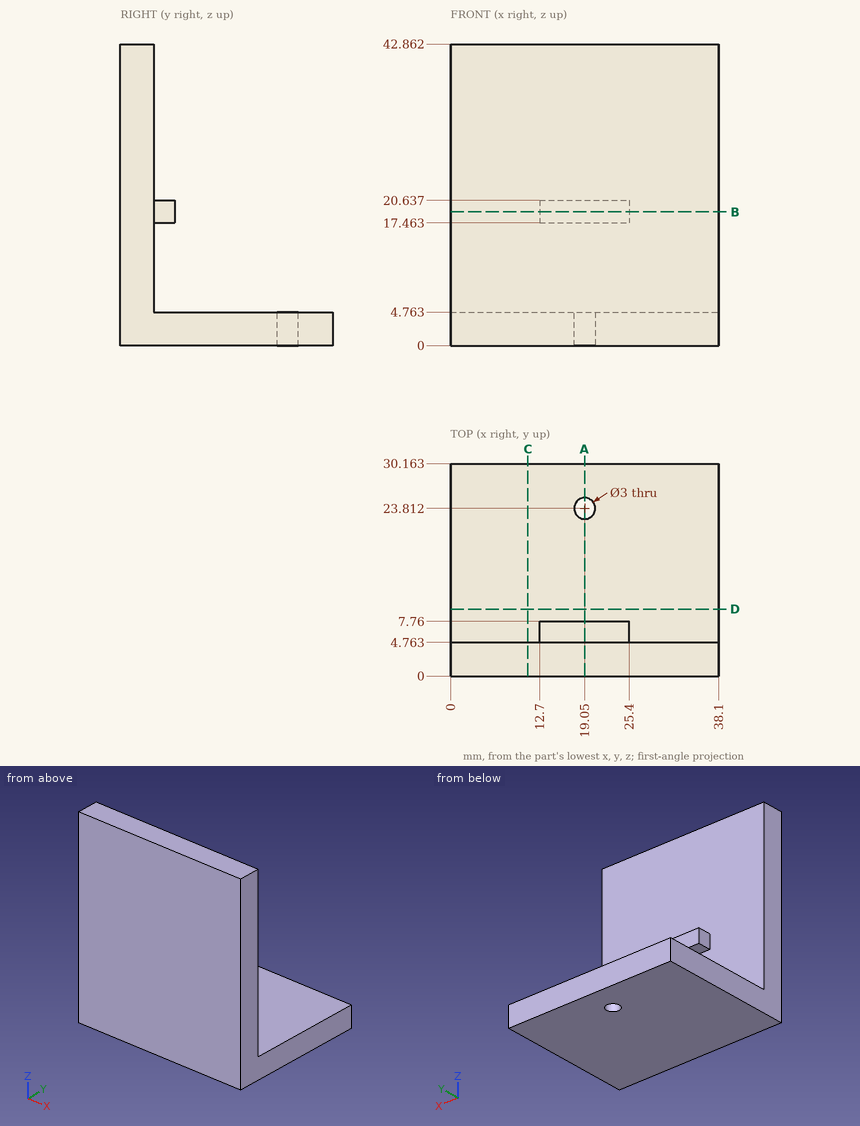
Can you work these out from the drawing? Everything is in mm from the part's minimum corner. Coordinates: 2 decimals unless noted, no trailing zeros. Loops run counter-clockwise (first coordinate to the right, second up) from the corner with the lowest first, then second, coordinate; pieces in that order, holes last. Notation, with made-up numbers: M 88.5,-37.5 L 97.5,-37.5 A23 ccw 97.5,-0.5 Z; hole C 24.25,67 d11. An arc over 180 degrees is marked long. Put each result on its own line as item: value. Start each with the question number.
(1) Suppose I cut it at B-B on z = 19. Please give me the cut outline in (x, y).
(2) I need wall thicknesses on line 1 (Y direction, x = 19.05, z = 3.75); line 2 (Y direction, x = 12.5, z = 31). Which ranges of each line are inside material? Lowest first, please. Write a range as from..to.
(3) Will these pins go through, and if not, where does the flat tip stop? P1, Ø8, axis at x = 11.5, y = 9, coming from the +Z side; P2, Ø3.5, axis at x = 22, z = 18.5, coming from the +Y side; P3, Ø12.5, axis at x = 17, y = 22, coming from the +Z side; P4, Ø2.5, axis at x = 19.05, y = 23.81, coming from the +Z side (3 decimals).
(4) Suppose I cut it at D-D on y = 9.5. Please give me the cut outline in (x, z).
(5) Suppose I cut it at A-A on x = 19.05. Please give me the cut outline in (y, z).
(6) Suppose I cut it at C-C on x = 11. Please give me the cut outline in (y, z).
Solutions:
1. outline: M 0,0 L 38.1,0 L 38.1,4.76 L 25.4,4.76 L 25.4,7.76 L 12.7,7.76 L 12.7,4.76 L 0,4.76 Z
2. line 1: y = 0..22.31, 25.31..30.16
2. line 2: y = 0..4.76
3. P1: stops at z = 20.64
3. P2: stops at y = 7.76
3. P3: stops at z = 4.76
3. P4: passes through
4. outline: M 0,0 L 38.1,0 L 38.1,4.76 L 0,4.76 Z
5. outline: M 0,0 L 22.31,0 L 22.31,4.76 L 4.76,4.76 L 4.76,17.46 L 7.76,17.46 L 7.76,20.64 L 4.76,20.64 L 4.76,42.86 L 0,42.86 Z; M 25.31,0 L 30.16,0 L 30.16,4.76 L 25.31,4.76 Z
6. outline: M 0,0 L 30.16,0 L 30.16,4.76 L 4.76,4.76 L 4.76,42.86 L 0,42.86 Z
